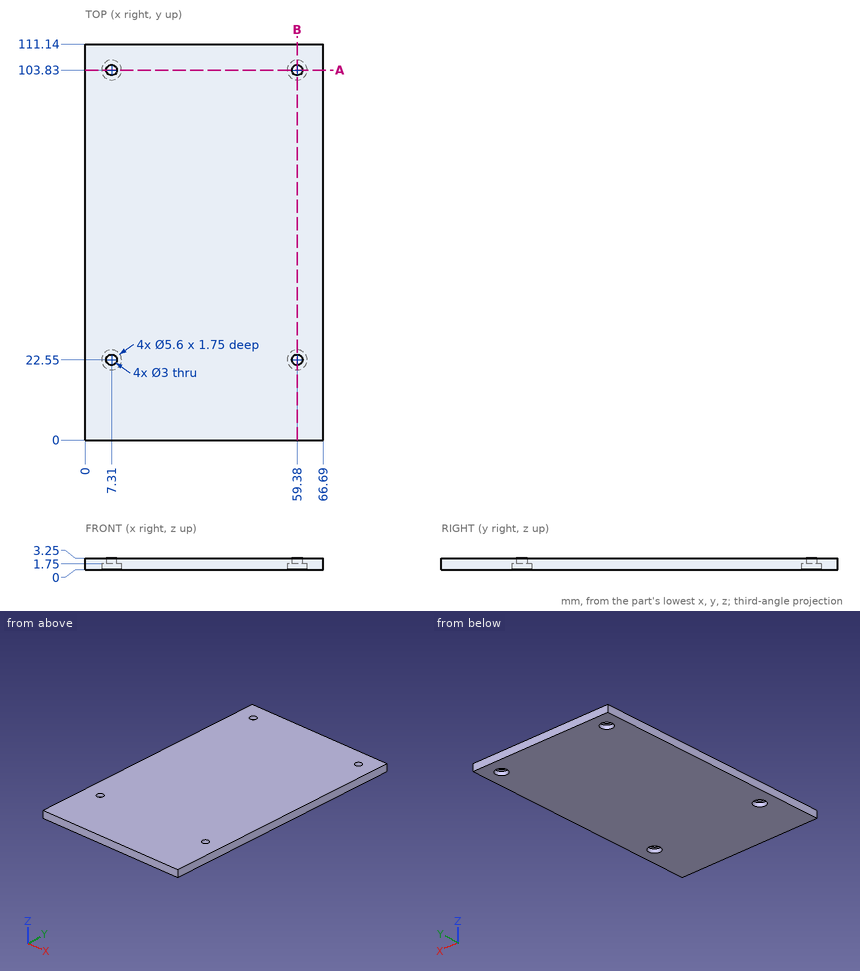
Geometry check sheet. Reference: drawing and pictorial views, mm from the part's lowest x, y, z. Coordinates: 2 decimals unless noted, no trailing zeros. Write each loop counter-clockwise with the first axis right and the second up, starting at its lowest first coordinate (ties: lowest second). Pieces come first, ordered by that corner, then holes. Notation, with made-up numbers: M 23.5,47 L 36.5,47 A15 cw 36.5,52 Z; hole C 60,-16 d5. An arc over 180 degrees is marked long. Write item = value, one per line. Start each with the question number.
1. Thickness scan on probe 1 along Y at (x, z) = (7.31, 0.7); probe 2 along X at (y, z) = (103.83, 2.5); probe 3 along Y at (x, z) = (59.38, 2.95). Record the ranges inside material, lowest first.
2. Sectioned sample at B-B (x = 59.38). Record the cut outline in (y, z), then the cut area to 3 significant figures.
3. Go/stop test with a flat-tipped pin: pin 1 (3 mm diameter, centred on x = 59, y = 105, fed in from -Z). Record where the tip stops, or that it passes through.
4. Sectioned sample at A-A (y = 103.83). Record the cut outline in (x, z), then the cut area to 3 significant figures.
The answers:
q1.probe_1 = 0 to 19.75, 25.35 to 101.03, 106.63 to 111.14
q1.probe_2 = 0 to 5.81, 8.81 to 57.88, 60.88 to 66.69
q1.probe_3 = 0 to 21.05, 24.05 to 102.33, 105.33 to 111.14
q2.outline = M 0,0 L 19.75,0 L 19.75,1.75 L 21.05,1.75 L 21.05,3.25 L 0,3.25 Z; M 24.05,1.75 L 25.35,1.75 L 25.35,0 L 101.03,0 L 101.03,1.75 L 102.33,1.75 L 102.33,3.25 L 24.05,3.25 Z; M 105.33,1.75 L 106.63,1.75 L 106.63,0 L 111.14,0 L 111.14,3.25 L 105.33,3.25 Z
q2.area = 333 mm²
q3.pin_1 = 1.75
q4.outline = M 0,0 L 4.51,0 L 4.51,1.75 L 5.81,1.75 L 5.81,3.25 L 0,3.25 Z; M 8.81,1.75 L 10.11,1.75 L 10.11,0 L 56.58,0 L 56.58,1.75 L 57.88,1.75 L 57.88,3.25 L 8.81,3.25 Z; M 60.88,1.75 L 62.18,1.75 L 62.18,0 L 66.69,0 L 66.69,3.25 L 60.88,3.25 Z
q4.area = 188 mm²
